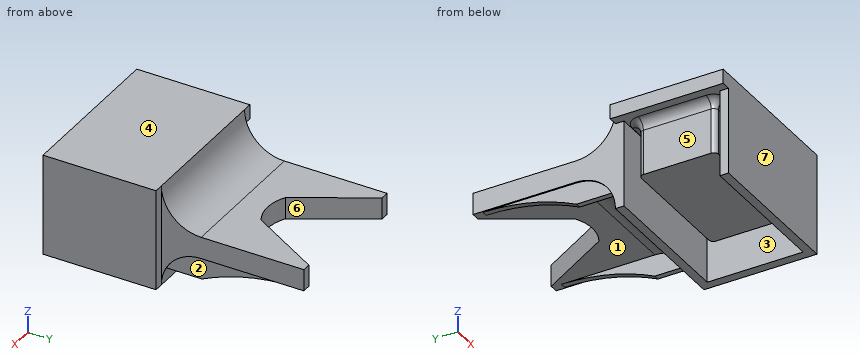
Autodesk Fusion 360 part; units mm, degrees
ref_plane "WorkPlane1" through (0, 0, -38) normal (0, 0, 1) x (1, 0, 0)
sketch "Sketch1" plane through (0, 0, -38) normal (0, 0, 1) x (1, 0, 0)
  line L0 (-34.25, -21.25) -> (34.25, -21.25)
  line L1 (34.25, -21.25) -> (34.25, 21.25)
  line L2 (34.25, 21.25) -> (-34.25, 21.25)
  line L3 (-34.25, 21.25) -> (-34.25, -21.25)
extrude "Extrude1" add sketch "Sketch1" along normal blind 30
fillet "Fillet1" radius 2.5 4 edges at (-34.25, 21.25, -23) (34.25, 21.25, -23) (34.25, -21.25, -23) (-34.25, -21.25, -23)
ref_plane "WorkPlane2" through (0, 0, -8) normal (0, 0, 1) x (1, 0, 0)
sketch "Sketch2" plane through (0, 0, -8) normal (0, 0, 1) x (1, 0, 0)
  line L0 (-44.25, -31.25) -> (44.25, -31.25)
  line L1 (44.25, -31.25) -> (44.25, 31.25)
  line L2 (44.25, 31.25) -> (-44.25, 31.25)
  line L3 (-44.25, 31.25) -> (-44.25, -31.25)
extrude "Extrude2" add sketch "Sketch2" along normal blind 8
ref_plane "WorkPlane3" through (0, 0, -38) normal (0, 0, 1) x (1, 0, 0)
sketch "Sketch3" plane through (0, 0, -38) normal (0, 0, 1) x (1, 0, 0)
  line L0 (-44.25, -31.25) -> (44.25, -31.25)
  line L1 (44.25, -31.25) -> (44.25, 31.25)
  line L2 (44.25, 31.25) -> (-44.25, 31.25)
  line L3 (-44.25, 31.25) -> (-44.25, -31.25)
  line L4 (-39.25, -26.5) -> (39.25, -26.5)
  line L5 (39.25, -26.5) -> (39.25, 26.5)
  line L6 (39.25, 26.5) -> (-39.25, 26.5)
  line L7 (-39.25, 26.5) -> (-39.25, -26.5)
extrude "Extrude3" add sketch "Sketch3" along normal blind 30
ref_plane "WorkPlane4" through (0, 0, -34) normal (0, 0, 1) x (1, 0, 0)
sketch "Sketch4" plane through (0, 0, -34) normal (0, 0, 1) x (1, 0, 0)
  line L0 (-44.25, 26.5) -> (44.25, 26.5)
  line L1 (44.25, 26.5) -> (44.25, 110)
  line L2 (44.25, 110) -> (-44.25, 110)
  line L3 (-44.25, 110) -> (-44.25, 26.5)
extrude "Extrude4" add sketch "Sketch4" along normal blind 12
sketch "Sketch5" plane through (0, 0, -34) normal (0, 0, 1) x (1, 0, 0)
  line L0 (-34.547, 110) -> (-11.5, 70.0814)
  arc A0 (-11.5, 70.0814) -> (11.5, 70.0814) centre (0, 90) ccw
  line L1 (11.5, 70.0814) -> (34.547, 110)
  line L2 (34.547, 110) -> (34.547, 115)
  line L3 (34.547, 115) -> (-34.547, 115)
  line L4 (-34.547, 115) -> (-34.547, 110)
extrude "Extrude5" cut sketch "Sketch5" along normal blind 12
fillet "Fillet2" radius 5 64 edges at (33.5178, -20.5178, -8) (0, -21.25, -8) (-33.5178, -20.5178, -8) (-34.25, 0, -8) (-33.5178, 20.5178, -8) (0, 21.25, -8) (33.5178, 20.5178, -8) (34.25, 0, -8) (34.25, 0, -8) (33.5178, 20.5178, -8) (0, 21.25, -8) (-33.5178, 20.5178, -8) (-34.25, 0, -8) (-33.5178, -20.5178, -8) (0, -21.25, -8) (33.5178, -20.5178, -8) (33.5178, 20.5178, -8) (34.25, 0, -8) (33.5178, -20.5178, -8) (0, -21.25, -8) (-33.5178, -20.5178, -8) (-34.25, 0, -8) (-33.5178, 20.5178, -8) (0, 21.25, -8) (0, 21.25, -8) (-33.5178, 20.5178, -8) (-34.25, 0, -8) (-33.5178, -20.5178, -8) (0, -21.25, -8) (33.5178, -20.5178, -8) (34.25, 0, -8) (33.5178, 20.5178, -8) (-33.5178, 20.5178, -8) (0, 21.25, -8) (33.5178, 20.5178, -8) (34.25, 0, -8) (33.5178, -20.5178, -8) (0, -21.25, -8) (-33.5178, -20.5178, -8) (-34.25, 0, -8) (-34.25, 0, -8) (-33.5178, -20.5178, -8) (0, -21.25, -8) (33.5178, -20.5178, -8) (34.25, 0, -8) (33.5178, 20.5178, -8) (0, 21.25, -8) (-33.5178, 20.5178, -8) (-33.5178, -20.5178, -8) (-34.25, 0, -8) (-33.5178, 20.5178, -8) (0, 21.25, -8) (33.5178, 20.5178, -8) (34.25, 0, -8) (33.5178, -20.5178, -8) (0, -21.25, -8) (0, -21.25, -8) (33.5178, -20.5178, -8) (34.25, 0, -8) (33.5178, 20.5178, -8) (0, 21.25, -8) (-33.5178, 20.5178, -8) (-34.25, 0, -8) (-33.5178, -20.5178, -8)
ref_plane "WorkPlane5" through (0, 0, -38) normal (0, 0, 1) x (1, 0, 0)
sketch "Sketch6" plane through (0, 0, -38) normal (0, 0, 1) x (1, 0, 0)
ref_plane "WorkPlane6" through (-39.25, 0, 0) normal (1, 0, 0) x (0, 1, 0)
sketch "Sketch8" plane through (-39.25, 0, 0) normal (1, 0, 0) x (0, 0, -1)
ref_plane "WorkPlane7" through (-39.25, 0, 0) normal (1, 0, 0) x (0, 1, 0)
sketch "Sketch9" plane through (-39.25, 0, 0) normal (1, 0, 0) x (0, 0, -1)
  line L0 (0, 31.25) -> (22, 31.25)
  line L1 (22, 31.25) -> (22, 53.25)
  arc A0 (0, 31.25) -> (22, 53.25) centre (0.0125, 53.2375) ccw
extrude "Extrude6" add sketch "Sketch9" along normal blind 83.5
ref_plane "WorkPlane8" through (0, 0, -38) normal (0, 0, 1) x (1, 0, 0)
sketch "Sketch10" plane through (0, 0, -38) normal (0, 0, 1) x (1, 0, 0)
  line L0 (-44.25, -31.25) -> (-39.25, -31.25)
  line L1 (-39.25, -31.25) -> (-39.25, 31.25)
  line L2 (-39.25, 31.25) -> (-44.25, 31.25)
  line L3 (-44.25, 31.25) -> (-44.25, -31.25)
extrude "Extrude7" cut sketch "Sketch10" along normal blind 30
ref_plane "WorkPlane9" through (0, 0, -56) normal (0, 0, 1) x (1, 0, 0)
sketch "Sketch11" plane through (0, 0, -56) normal (0, 0, 1) x (1, 0, 0)
  line L0 (-44.25, -31.25) -> (44.25, -31.25)
  line L1 (44.25, -31.25) -> (44.25, 31.25)
  line L2 (44.25, 31.25) -> (-44.25, 31.25)
  line L3 (-44.25, 31.25) -> (-44.25, -31.25)
  line L4 (-39.25, -26.5) -> (39.25, -26.5)
  line L5 (39.25, -26.5) -> (39.25, 26.5)
  line L6 (39.25, 26.5) -> (-39.25, 26.5)
  line L7 (-39.25, 26.5) -> (-39.25, -26.5)
extrude "Extrude8" add sketch "Sketch11" along normal blind 18
ref_plane "WorkPlane10" through (0, 0, -56) normal (0, 0, 1) x (1, 0, 0)
sketch "Sketch12" plane through (0, 0, -56) normal (0, 0, 1) x (1, 0, 0)
  line L0 (-44.25, -31.25) -> (-39.25, -31.25)
  line L1 (-39.25, -31.25) -> (-39.25, 31.25)
  line L2 (-39.25, 31.25) -> (-44.25, 31.25)
  line L3 (-44.25, 31.25) -> (-44.25, -31.25)
extrude "Extrude9" cut sketch "Sketch12" along normal blind 18
ref_plane "WorkPlane11" through (0, 0, -34) normal (0, 0, 1) x (1, 0, 0)
sketch "Sketch13" plane through (0, 0, -34) normal (0, 0, 1) x (1, 0, 0)
  line L0 (-44.25, 31.25) -> (-39.25, 31.25)
  line L1 (-39.25, 31.25) -> (-39.25, 110)
  line L2 (-39.25, 110) -> (-44.25, 110)
  line L3 (-44.25, 110) -> (-44.25, 31.25)
extrude "Extrude10" cut sketch "Sketch13" along normal blind 12
ref_plane "WorkPlane12" through (-39.25, 0, 0) normal (1, 0, 0) x (0, 1, 0)
sketch "Sketch14" plane through (-39.25, 0, 0) normal (1, 0, 0) x (0, 0, -1)
  line L0 (56, 31.25) -> (34, 31.25)
  line L1 (34, 31.25) -> (34, 53.25)
  arc A0 (34, 53.25) -> (56, 31.25) centre (55.9875, 53.2375) ccw
extrude "Extrude11" add sketch "Sketch14" along normal blind 83.5
ref_plane "WorkPlane13" through (0, 0, -46) normal (0, 0, 1) x (1, 0, 0)
sketch "Sketch15" plane through (0, 0, -46) normal (0, 0, 1) x (1, 0, 0)
  line L0 (-38.5, 31.25) -> (-35.5, 31.25)
  line L1 (-35.5, 31.25) -> (-35.5, 105)
  line L2 (-35.5, 105) -> (-38.5, 105)
  line L3 (-38.5, 105) -> (-38.5, 31.25)
  line L4 (35.5, 31.25) -> (38.5, 31.25)
  line L5 (38.5, 31.25) -> (38.5, 105)
  line L6 (38.5, 105) -> (35.5, 105)
  line L7 (35.5, 105) -> (35.5, 31.25)
extrude "Extrude12" add sketch "Sketch15" along normal blind 12
ref_plane "WorkPlane14" through (35.5, 0, 0) normal (1, 0, 0) x (0, 1, 0)
sketch "Sketch16" plane through (35.5, 0, 0) normal (1, 0, 0) x (0, 0, -1)
  arc A0 (34, 105) -> (46, 53.25) centre (151.5034, 104.9809) ccw
  line L0 (34, 105) -> (46, 105)
  line L1 (46, 105) -> (46, 53.25)
extrude "Extrude13" cut sketch "Sketch16" along normal blind 3
ref_plane "WorkPlane15" through (-38.5, 0, 0) normal (1, 0, 0) x (0, 1, 0)
sketch "Sketch17" plane through (-38.5, 0, 0) normal (1, 0, 0) x (0, 0, -1)
  arc A0 (34, 105) -> (46, 53.25) centre (151.5034, 104.9809) ccw
  line L0 (34, 105) -> (46, 105)
  line L1 (46, 105) -> (46, 53.25)
extrude "Extrude14" cut sketch "Sketch17" along normal blind 3
ref_plane "WorkPlane16" through (0, 0, -56) normal (0, 0, 1) x (1, 0, 0)
sketch "Sketch18" plane through (0, 0, -56) normal (0, 0, 1) x (1, 0, 0)
  line L0 (39.25, 31.25) -> (44.25, 31.25)
  line L1 (44.25, 31.25) -> (44.25, 110)
  line L2 (44.25, 110) -> (39.25, 110)
  line L3 (39.25, 110) -> (39.25, 31.25)
extrude "Extrude15" cut sketch "Sketch18" along normal blind 56
Can you work these out from the model? Positions are in its coordinate system, mm. Face numbers are marked on the shaded views. A direction names the side the tool comes from. Give positions to 0.01 mm unless a question says otherwise; leave off trailing zeros. Loops run counter-clockwise (first coordinate to the right, second up) from the corner with the lowest first, then second, coordinate; pieces in that order, holes last. Notation, with made-up numbers: M 88,-4 L 123,-4 A20 cw 123,32 Z; hole C 8.5,20 d7. An arc over 180 degrees is marked long. One line per item, written item: value.
1) Thinking about a two-plate mould opening in Y: for the marked faces 4, 5, 6 and 7, which applies, +Y half, -Y half, draft (parallel to the pull), parting line (faces both ways), or undercut?
Geometry check:
face 4: draft
face 5: undercut
face 6: +Y half
face 7: -Y half
2) Please list where these lines run through material, in increasing order: line 1 (Y direction, x = -15.5, z = -16); line 2 (X direction, y = 3, z = -19); line 3 (Y direction, x = 38.5, z = -26).
Geometry check:
line 1: y = -31.25 to -26.5, -21.25 to 21.25, 26.5 to 38.14
line 2: x = -34.25 to 34.25, 39.25 to 44.25
line 3: y = -31.25 to -26.5, 26.5 to 110
3) Imagine slicing it at A-A on z = -16.5. Write out the boundary of the cut face in (x, y).
Geometry check:
outline: M -39.25,-31.25 L 44.25,-31.25 L 44.25,31.25 L 39.25,31.25 L 39.25,38.69 L -39.25,38.69 L -39.25,26.5 L 39.25,26.5 L 39.25,-26.5 L -39.25,-26.5 Z; M -34.25,-18.75 A2.5 ccw -31.75,-21.25 L 31.75,-21.25 A2.5 ccw 34.25,-18.75 L 34.25,18.75 A2.5 ccw 31.75,21.25 L -31.75,21.25 A2.5 ccw -34.25,18.75 Z
4) On a 3-axis mill with a long thin cutter (end or side, diameter ignored), from which of +Z, -Z, +X, -X, +Y, -Y can I reach the whole of each face in a straight line? I mean the marked faces 1, 2 and 3. Say none if no direction works.
Geometry check:
face 1: -Z, +Y
face 2: -Z, +X, +Y
face 3: -Z
5) I'm going to push flat-ended pins straight in: pin 1 (1.5 mm diameter, centred on x = -42, z = -5.5, fed in from +Y); pin 2 (8 mm diameter, centred on x = 1, z = -9.5, fed in from +Y); pin 3 (3.5 mm diameter, centred on y = 66.5, z = -39, fed in from +X); pin 4 (10 mm diameter, centred on y = 75, z = -14, fed in from +X). Where does each tip first touch, or does it pass through?
Geometry check:
pin 1: stops at y = 31.25
pin 2: stops at y = 35.87
pin 3: stops at x = 38.5
pin 4: passes through
6) Imagine slicing it at B-B on y = 99. Write out the boundary of the cut face in (x, z).
Geometry check:
outline: M -39.25,-34 L -38.5,-34 L -38.5,-34.15 L -35.5,-34.15 L -35.5,-34 L -28.2,-34 L -28.2,-22 L -39.25,-22 Z; M 28.2,-34 L 35.5,-34 L 35.5,-34.15 L 38.5,-34.15 L 38.5,-34 L 39.25,-34 L 39.25,-22 L 28.2,-22 Z
7) Imagine slicing it at D-D on y = 76. Write out the boundary of the cut face in (x, z), and give its area (3 significant figures).
Geometry check:
outline: M -39.25,-34 L -38.5,-34 L -38.5,-37.63 L -35.5,-37.63 L -35.5,-34 L -14.92,-34 L -14.92,-22 L -39.25,-22 Z; M 14.92,-34 L 35.5,-34 L 35.5,-37.63 L 38.5,-37.63 L 38.5,-34 L 39.25,-34 L 39.25,-22 L 14.92,-22 Z
area: 606 mm²
